from build123d import *

# Parameters (mm, degrees)
SKETCH1_W           = 45
SKETCH1_H           = 20
BOSS_EXTRUDE1_DEPTH = 1.54
SKETCH2_R           = 8
BOSS_EXTRUDE2_DEPTH = 13
BOSS_EXTRUDE3_DEPTH = 4
SKETCH4_W           = 8.9
SKETCH4_H           = 4
SKETCH4_W_2         = 4
SKETCH4_H_2         = 8.9
BOSS_EXTRUDE4_DEPTH = 3.5


with BuildPart() as part:
    # Sketch1 → Boss-Extrude1 (new body)
    with BuildSketch(Plane(origin=(0, 0, 0), x_dir=(1, 0, 0), z_dir=(0, 1, 0))):
        Rectangle(SKETCH1_W, SKETCH1_H)
    extrude(amount=BOSS_EXTRUDE1_DEPTH)

    # Sketch2 → Boss-Extrude2 (add)
    with BuildSketch(Plane(origin=(0, 1.54, 0), x_dir=(1, 0, 0), z_dir=(0, 1, 0))):
        with Locations(Location((-13.25, 0, 0), (0, 0, 90))):
            Circle(SKETCH2_R)
        with Locations(Location((13.25, 0, 0), (0, 0, 90))):
            Circle(SKETCH2_R)
    extrude(amount=BOSS_EXTRUDE2_DEPTH)

    # Sketch3 → Boss-Extrude3 (add)
    with BuildSketch(Plane(origin=(0, 1.54, 0), x_dir=(1, 0, 0), z_dir=(0, 1, 0))):
        with BuildLine():
            Line((-4.3864516, 9), (4.3864516, 9))
            ThreePointArc((4.3864516, 9), (6.3864516, 7), (4.3864516, 5))
            Line((4.3864516, 5), (-4.3864516, 5))
            ThreePointArc((-4.3864516, 5), (-6.3864516, 7), (-4.3864516, 9))
        make_face()
    extrude(amount=BOSS_EXTRUDE3_DEPTH)

    # Sketch4 → Boss-Extrude4 (add)
    with BuildSketch(Plane(origin=(0, 0, 0), x_dir=(1, 0, 0), z_dir=(0, 1, 0))):
        Rectangle(SKETCH4_W, SKETCH4_H)
        with Locations((16.25, -0.384163824)):
            Rectangle(SKETCH4_W, SKETCH4_H)
        with Locations((-17.9, -1.55)):
            Rectangle(SKETCH4_W_2, SKETCH4_H_2)
    extrude(amount=-BOSS_EXTRUDE4_DEPTH)


solid = part.part
Can you work these out from the model? Positions are in its coordinate system, mm. A direction names the side the tool comes from. Give positions to 0.01 mm unless a question says otherwise; leave off trailing zeros. Order: outer loops, then holes, each group sorted by start corner. A loop starts at its lowest first (then second) coordinate and runs counter-clockwise, first axis right, second up. Notation, with made-up numbers: M 72.5,43 L 97.5,43 A31 cw 97.5,72 Z; hole C -24.5,-21.5 d10. An arc over 180 degrees is marked long. Use one line per item in the form item = value. Start each with the question number.
Item 1: Will these pins go through, and if not, where does the flat tip stop? pin 1 Ø6 at (x, z) = (-9.5, 0) entering from -Y; pin 2 Ø1 at (x, y) = (1.5, -1) entering from +Z; pin 3 Ø1.5 at (y, z) = (8.5, -5.5) entering from -X.
Item 2: If I drill on line 1 along X through (y, z) = (-2, 0); line 2 along Y through (x, z) = (-14.5, -8.5); line 3 along X through (y, z) = (6, 0), over which ranges is the centre line in solid material (lowest first)?
Item 3: For faces 1 (the flat face through (0, -2, -2)), 2 (the flat face through (-18, -2, -2.9)), 3 (the cylindrical face through (21.06, 7.95, 1.73)), 4 (the flat face through (-15.9, -2, 2)), which set-ups out of +Z, -Z, +X, -X, +Y, -Y let a thin tool reach every point of the face, with its end or its side?
Item 4: If we section it at C-C (x = 0.5): Write out the boundary of the cut face in (y, z), then the cut area to 3 significant figures.
Item 5: If we section it at A-A (z = 0): Write out the boundary of the cut face in (x, y).
Item 6: If we section it at B-B (y = 2.75): Write out the boundary of the cut face in (x, z), then the cut area to 3 significant figures.
Item 7: If we section it at D-D (y = 11.5): Write out the boundary of the cut face in (x, z), then the cut area to 3 significant figures.
Item 8: We'd pull the mould along Z, two halves only. Please class faces 5 (the cylindrical face through (6.386, 3.512, -7.044)), 6 (the flat face through (0, 5.54, -7)), 7 (the flat face through (0, 4, -5)), 8 (the flat face through (0, 1, -10)): +Z half, -Z half, draft (parallel to the pull), parting line (faces both ways), or undercut.
Outcome:
q1.pin_1 = 0
q1.pin_2 = 2
q1.pin_3 = -19.69
q2.line_1 = -19.9 to -15.9, -4.45 to 4.45, 11.8 to 20.7
q2.line_2 = 0 to 1.54
q2.line_3 = -21.25 to -5.25, 5.25 to 21.25
q3.face_1 = -Z, +X, -Y
q3.face_2 = -Z, +X, -X, -Y
q3.face_3 = +Y
q3.face_4 = +Z, -Z, -Y
q4.outline = M -3.5,-2 L 0,-2 L 0,-10 L 1.54,-10 L 1.54,-9 L 5.54,-9 L 5.54,-5 L 1.54,-5 L 1.54,10 L 0,10 L 0,2 L -3.5,2 Z
q4.area = 60.8 mm2
q5.outline = M -22.5,0 L -19.9,0 L -19.9,-3.5 L -15.9,-3.5 L -15.9,0 L -4.45,0 L -4.45,-3.5 L 4.45,-3.5 L 4.45,0 L 11.8,0 L 11.8,-3.5 L 20.7,-3.5 L 20.7,0 L 22.5,0 L 22.5,1.54 L 21.25,1.54 L 21.25,14.54 L 5.25,14.54 L 5.25,1.54 L -5.25,1.54 L -5.25,14.54 L -21.25,14.54 L -21.25,1.54 L -22.5,1.54 Z
q6.outline = C -13.25,0 d16; M -4.39,-9 L 4.39,-9 A2 ccw 4.39,-5 L -4.39,-5 A2 ccw Z; C 13.25,0 d16
q6.area = 450 mm2
q7.outline = C -13.25,0 d16; C 13.25,0 d16
q7.area = 402 mm2
q8.face_5 = undercut
q8.face_6 = draft
q8.face_7 = +Z half
q8.face_8 = -Z half
